Verification items for the finished model (mm, model axes). A direction names the side the tool comes from. Give positions to 0.01 mm unless a question says otherwise; leave off trailing zeros. Loops run counter-clockwise (first coordinate to the right, second up) from the corner with the lowest first, then second, coordinate; pieces in that order, holes last. Notation, with made-up numbers: (-18, 17) - (32, 17) arc R21 ccw to (32, 23) - close; hole circle Ø6 at (70.5, 36). An arc over 180 degrees is marked (long way). Use one line per item in the form item = value.
```python
from build123d import *

# Parameters (mm, degrees)
BOSS_EXTRUDE1_DEPTH = 3.2
CUT_EXTRUDE1_START  = -2.25739
CUT_EXTRUDE1_DEPTH  = 4.51476888
SKETCH6_W           = 6
SKETCH6_H           = 16.9095993
BOSS_EXTRUDE2_DEPTH = 3
SKETCH7_OUTSIDE_W   = 20.212
SKETCH7_OUTSIDE_H   = 20.212
SKETCH7_OUTSIDE_W_2 = 6
SKETCH7_OUTSIDE_H_2 = 4
CUT_EXTRUDE2_DEPTH  = 8
FILLET1_R           = 1
FILLET2_R           = 0.5
SKETCH8_R           = 1
CUT_EXTRUDE3_DEPTH  = 14


# Read off the part's stored shape, not the designer's step: Cut-Extrude1
with BuildPart() as part:
    # Sketch1 → Revolve1 (revolve)
    with BuildSketch(Plane(origin=(0, 0, 0), x_dir=(1, 0, 0), z_dir=(0, 1, 0))):
        with BuildLine():
            Line((0, 5.7), (0, -5.7))
            ThreePointArc((0, -5.7), (5.7, 0), (0, 5.7))
        make_face()
    revolve(axis=Axis((0, 0, 14.54011976), (0, 0, -1)))

    # Sketch2 → Boss-Extrude1 (add, symmetric)
    with BuildSketch(Plane(origin=(0, 0, 0), x_dir=(0, 0, -1), z_dir=(1, 0, 0))):
        with BuildLine():
            Line((-3.95, 0), (3.95, 0))
            Line((3.95, 0), (3.95, -8.3))
            ThreePointArc((3.95, -8.3), (-0.079654203, -7.901360118), (-3.95, -6.710792959))
            Line((-3.95, -6.710792959), (-3.95, 0))
        make_face()
    extrude(amount=BOSS_EXTRUDE1_DEPTH, both=True)

    # Sketch3 → Revolve2 (revolve)
    with BuildSketch(Plane(origin=(0, 0, 0), x_dir=(0, 0, -1), z_dir=(1, 0, 0)), mode=Mode.PRIVATE) as revolve2_sk:
        Polygon((0.95, -7.401163559), (0.95, -11.652192734), (3.2, -11.652192734), (3.95, -7.401163559), align=None)
    revolve(revolve2_sk.sketch.rotate(Axis((0, -11.652192734, -0.95), (0, 1, 0)), 45.250719205), axis=Axis((0, -11.652192734, -0.95), (0, 1, 0)))

    # Cut-Extrude1 outline → Cut-Extrude1 (cut)
    with BuildSketch(Plane(origin=(0, 0, 0), x_dir=(0, 0, -1), z_dir=(1, 0, 0)).offset(CUT_EXTRUDE1_START)):
        with BuildLine():
            Line((-3, -11.652192734), (1.275092895, -11.652192734))
            ThreePointArc((1.275092895, -11.652192734), (-0.058768815, -11.464467118), (-1.379872872, -11.201575434))
            Line((-1.379872872, -11.201575434), (-3, -10.831225258))
            Line((-3, -10.831225258), (-3, -11.652192734))
        make_face()
    extrude(amount=CUT_EXTRUDE1_DEPTH, mode=Mode.SUBTRACT)

    # Sketch6 → Boss-Extrude2 (add, symmetric)
    with BuildSketch(Plane(origin=(0, 0, 0), x_dir=(0, 0, -1), z_dir=(1, 0, 0))):
        with Locations((0, 9.893007616)):
            Rectangle(SKETCH6_W, SKETCH6_H)
    extrude(amount=BOSS_EXTRUDE2_DEPTH, both=True)

    # Sketch7 outside → Cut-Extrude2 (cut)
    with BuildSketch(Plane(origin=(0, 18.347807266, 0), x_dir=(1, 0, 0), z_dir=(0, 1, 0))):
        Rectangle(SKETCH7_OUTSIDE_W, SKETCH7_OUTSIDE_H)
        Rectangle(SKETCH7_OUTSIDE_W_2, SKETCH7_OUTSIDE_H_2, mode=Mode.SUBTRACT)
    extrude(amount=-CUT_EXTRUDE2_DEPTH, mode=Mode.SUBTRACT)

    # Fillet1
    fillet1_edges = [part.edges().sort_by_distance(p)[0] for p in [
        (-3, 7.077190264, 3),
        (3, 7.077190264, 3),
        (-3, 7.077190264, -3),
        (3, 7.077190264, -3),
        (-3, 14.347807266, -2),
        (-3, 14.347807266, 2),
        (3, 14.347807266, -2),
        (3, 14.347807266, 2),
    ]]
    fillet(fillet1_edges, radius=FILLET1_R)

    # Fillet2
    fillet2_edges = [part.edges().sort_by_distance(p)[0] for p in [
        (-3.2, -4.644533788, 3.95),
        (3.2, -4.644533788, 3.95),
        (3.2, -5.439137308, -3.95),
        (-3.2, -5.439137308, -3.95),
    ]]
    fillet(fillet2_edges, radius=FILLET2_R)

    # Sketch8 → Cut-Extrude3 (cut)
    with BuildSketch(Plane(origin=(0, 18.347807266, 0), x_dir=(1, 0, 0), z_dir=(0, 1, 0))):
        with Locations(Location((0, 0, 0), (0, 0, 270))):
            Circle(SKETCH8_R)
    extrude(amount=-CUT_EXTRUDE3_DEPTH, mode=Mode.SUBTRACT)


solid = part.part
```
1. Section check D-D, the plane x = 4.75. Record the cut outline in (y, z).
Result set:
outline = circle Ø6.3 at (0, 0)
2. Section check A-A, the plane y = 7. Record the cut outline in (x, z), then the cut area to 3 significant figures.
Result set:
outline = (-3, -2) arc R1 ccw to (-2, -3) - (2, -3) arc R1 ccw to (3, -2) - (3, 2) arc R1 ccw to (2, 3) - (-2, 3) arc R1 ccw to (-3, 2) - close; hole circle Ø2 at (0, 0)
area = 32.0 mm²
3. Scan lines: probe 1 along X at (y, z) = (9.5, 0); probe 2 along Z at (x, y) = (1.25, 8); probe 3 along Y at (x, z) = (2, -0.5). Record each from-to range of solid material in increasing order.
Result set:
probe_1 = -3 to -1, 1 to 3
probe_2 = -3 to 3
probe_3 = -11.55 to 18.35
4. Section check C-C, the plane y = 2.5. Record the cut outline in (x, z) (1 decimal).
Result set:
outline = circle Ø10.2 at (0, 0)
5. Tool access check on faces 1 (the cylindrical face through (-2.699, 7.328, 2.715)), 2 (the cylindrical face through (2.699, 7.328, 2.715)), 3 (the cylindrical face through (2.715, 7.328, -2.699)), 4 (the cylindrical face through (0.045, -7.212, 2.634)). Record the directions out of +Z, -Z, +X, -X, +Y, -Y that give a thin tool (end or side, any length) a straight path to the whole face; none if there is none.
Result set:
face_1 = +Z, -X, +Y
face_2 = +Z, +X, +Y
face_3 = -Z, +X, +Y
face_4 = -Y
6. Draft check along X on faces 5 (the flat face through (-3, 10, 0)), 6 (the flat face through (0, -6, -3.95)), 7 (the cylindrical face through (-1, 11, 0)). Enter one of: released by +X, released by -X, zero draft, split by the parting line, or undercut.
Result set:
face_5 = released by -X
face_6 = zero draft
face_7 = undercut
7. Section check B-B, the plane x = 0. Record the cut outline in (y, z), then the cut area to 3 significant figures.
Result set:
outline = (-11.65, -3.2) - (-8.3, -3.79) arc R20.3 ccw to (-8.3, -3.95) - (-4.11, -3.95) arc R5.7 ccw to (4.85, -3) - (10.35, -3) - (10.35, -2) - (18.35, -2) - (18.35, -1) - (4.35, -1) - (4.35, 1) - (18.35, 1) - (18.35, 2) - (10.35, 2) - (10.35, 3) - (4.85, 3) arc R5.7 ccw to (-4.11, 3.95) - (-6.71, 3.95) arc R20.3 ccw to (-7.4, 2.05) - (-11.2, 1.38) arc R23.8 ccw to (-11.65, -1.28) - close
area = 174 mm²
8. Depth check by flat-ended pin: pin 1 Ø1 at (x, y) = (-0.5, 3) entering from +Z; pin 2 Ø4 at (y, z) = (-5, -1) entering from +X; pin 3 Ø3 at (x, y) = (-4, 8) entering from +Z. Enter the tip coordinate at first touch or a pass-through.
Result set:
pin_1 = 5.1
pin_2 = 4.78
pin_3 = 2.87
